Design review of the part built by this model. Coordinates are the model's own, in mm. A direction names the side the tool comes from. Coordinates: 2 decimals unless noted, no trailing zeros. Write each loop counter-clockwise with the first axis right and the second up, starting at its lowest first coordinate (ties: lowest second). Pieces come first, ordered by that corner, then holes.
```python
from build123d import *

# Parameters (mm, degrees)
CROQUIS1_W              = 23
CROQUIS1_H              = 12
SALIENTE_EXTRUIR1_DEPTH = 18
CROQUIS2_W              = 15
CROQUIS2_H              = 9
CORTAR_EXTRUIR1_DEPTH   = 20
CROQUIS3_W              = 1.1
CROQUIS3_H              = 9
CORTAR_EXTRUIR2_DEPTH   = 24
CROQUIS4_R              = 1.5
CORTAR_EXTRUIR3_DEPTH   = 4


with BuildPart() as part:
    # Croquis1 → Saliente-Extruir1 (new body)
    with BuildSketch(Plane.XY):
        Rectangle(CROQUIS1_W, CROQUIS1_H)
    extrude(amount=SALIENTE_EXTRUIR1_DEPTH)

    # Croquis2 → Cortar-Extruir1 (cut)
    with BuildSketch(Plane(origin=(11.5, 0, 0), x_dir=(0, 0, -1), z_dir=(1, 0, 0))):
        with Locations((-7.5, -1.5)):
            Rectangle(CROQUIS2_W, CROQUIS2_H)
    extrude(amount=-CORTAR_EXTRUIR1_DEPTH, mode=Mode.SUBTRACT)

    # Croquis3 → Cortar-Extruir2 (cut, through all)
    with BuildSketch(Plane.ZY.offset(11.5)):
        with Locations((14.45, -1.5)):
            Rectangle(CROQUIS3_W, CROQUIS3_H)
    extrude(amount=-CORTAR_EXTRUIR2_DEPTH, mode=Mode.SUBTRACT)

    # Croquis4 → Cortar-Extruir3 (cut, through all)
    with BuildSketch(Plane(origin=(0, 0, 15), x_dir=(-1, 0, 0), z_dir=(0, 0, -1))):
        with Locations((-5.5, -1.5)):
            Circle(CROQUIS4_R)
        with Locations((3.5, -1.5)):
            Circle(CROQUIS4_R)
    extrude(amount=-CORTAR_EXTRUIR3_DEPTH, mode=Mode.SUBTRACT)


solid = part.part
```
(1) Wall thickness on line 1 (Y direction, x = -3.5, z = 16.5); line 2 (X direction, y = -2, z = 16); line 3 (Y direction, x = -5, z = 7): over which ranges is each line inside the solid? List them lowest first.
(2) Consider section D-D (z = 16.25). Give the boundary of the cut face in (x, y), plus the area to 3 significant figures.
(3) Consider section A-A (y = -1.5). Give the boundary of the cut face in (x, z).
(4) Consider section B-B (y = -4.75). Give the boundary of the cut face in (x, z).
(5) Mouldability with a two-part tool opening along X and no side actions: class faces 1 (the flat face through (0, 0, 18)), 2 (the cylindrical face through (-4.886, -2.075, 16.479)), 3 (the flat face through (-11.5, 0, 9)) as +X half, -X half, draft (parallel to the pull), parting line (faces both ways), or undercut.
(6) For faces 4 (the flat face through (-8.5, -1, 7)), 5 (the flat face through (-10, -2, 13.9)), 6 (the cylindrical face through (6.7, -2.4, 16.5)), list the 3-axis set-ups (+Z, -Z, +X, -X, +Y, -Y) from which the entire face can be reached by the end or side of a thin tool; tool diameter is ignored.
(7) Consider section C-C (x = -3.5). Give the boundary of the cut face in (y, z), plus the area to 3 significant figures.
(8) Insertion check: pin 1 Ø5 at (x, z) = (-1, 14.5) entering from -Y; pin 2 Ø4.5 at (y, z) = (0.5, 10) entering from +X; pin 3 Ø3 at (x, y) = (6.5, 1) entering from -Z; pin 4 Ø8 at (x, z) = (-1, 7.5) entering from -Y. Each pin has a flat end and moves straight along its axis. Give the tip position at first contact, or say it passes through.
Results:
1. line 1: y = -6 to -3, 0 to 6
1. line 2: x = -11.5 to -4.91, -2.09 to 4.09, 6.91 to 11.5
1. line 3: y = 3 to 6
2. outline: (-11.5, -6) - (11.5, -6) - (11.5, 6) - (-11.5, 6) - close; hole circle Ø3 at (-3.5, -1.5); hole circle Ø3 at (5.5, -1.5)
2. area: 262 mm2
3. outline: (-11.5, 0) - (-8.5, 0) - (-8.5, 13.9) - (-11.5, 13.9) - close; (-11.5, 15) - (-5, 15) - (-5, 18) - (-11.5, 18) - close; (-2, 15) - (4, 15) - (4, 18) - (-2, 18) - close; (7, 15) - (11.5, 15) - (11.5, 18) - (7, 18) - close
4. outline: (-11.5, 0) - (-8.5, 0) - (-8.5, 13.9) - (-11.5, 13.9) - close; (-11.5, 15) - (11.5, 15) - (11.5, 18) - (-11.5, 18) - close
5. face 1: draft
5. face 2: undercut
5. face 3: -X half
6. face 4: -Z, +X, -Y
6. face 5: +X, -X, -Y
6. face 6: +Z, -Z
7. outline: (-6, 15) - (-3, 15) - (-3, 18) - (-6, 18) - close; (0, 15) - (3, 15) - (3, 0) - (6, 0) - (6, 18) - (0, 18) - close
7. area: 72.0 mm2
8. pin 1: stops at y = -6
8. pin 2: stops at x = -8.5
8. pin 3: stops at z = 15
8. pin 4: stops at y = 3
